Build history of the part. All positions in model axes, mm. Coordinates: 2 decimals unless noted, no trailing zeros. Order: outer loops, then holes, each group sorted by start corner. A loop starts at its lowest first (then second) coordinate and runs counter-clockwise, first axis right, second up. Notation, with made-up numbers: (42.5, 27) - (88.5, 27) arc R19 cw to (88.5, 49) - close; hole circle Ø9 at (48.5, 2). An arc over 180 degrees is marked (long way). Write each question's results on one line, items separated by ' | '.
from build123d import *

# Parameters (mm, degrees)
SKETCH1_W           = 2.87
SKETCH1_H           = 12.02
BOSS_EXTRUDE1_DEPTH = 2
CUT_EXTRUDE1_REACH  = 14.02


with BuildPart() as part:
    # Sketch1 → Boss-Extrude1 (new body)
    with BuildSketch(Plane.XY):
        with Locations((0, 6.01)):
            Rectangle(SKETCH1_W, SKETCH1_H)
    extrude(amount=BOSS_EXTRUDE1_DEPTH)

    # Sketch2 → Cut-Extrude1 (cut, up to next)
    with BuildSketch(Plane.XZ, mode=Mode.PRIVATE) as cut_extrude1_sk1:
        Polygon((0, -1.665063509), (1.25, 0.5), (-1.25, 0.5), align=None)
    cut_extrude1_tool1 = extrude(cut_extrude1_sk1.sketch, amount=-CUT_EXTRUDE1_REACH, mode=Mode.PRIVATE) & part.part
    add(cut_extrude1_tool1.solids().sort_by_distance((0, 0, -0.221688))[0], mode=Mode.SUBTRACT)


solid = part.part
1. Band-saw the part on A-A on z = 0.2. Give the cut face in (x, y) (3 decimals), then the cut area to 3 significant figures.
Solved:
outline: (-1.435, 0) - (-1.077, 0) - (-1.077, 12.02) - (-1.435, 12.02) - close; (1.077, 0) - (1.435, 0) - (1.435, 12.02) - (1.077, 12.02) - close | area: 8.61 mm2
2. Band-saw the part on B-B on y = 6.75. Give the cut face in (x, z) (3 decimals), then the cut area to 3 significant figures.
Solved:
outline: (-1.435, 0) - (-0.961, 0) - (-1.25, 0.5) - (1.25, 0.5) - (0.961, 0) - (1.435, 0) - (1.435, 2) - (-1.435, 2) - close | area: 4.63 mm2
3. Probe line 1 (Z direction, x = -0.3, y = 5.5); line 2 (Z direction, x = -1.1, y = 10.5); line 3 (X direction, y = 7.75, z = 0.1) (3 decimals). List the from-to ranges inside material, lowest first.
Solved:
line 1: z = 0.5 to 2 | line 2: z = 0 to 0.24, 0.5 to 2 | line 3: x = -1.435 to -1.019, 1.019 to 1.435
4. Two-plate mould, pull along Z, no slides. Class faces 1 (the face through (0, 0, 1)), 2 (the face through (0, 6, 0.5)), 3 (the face through (0, 6, 2)): +Z half, -Z half, draft (parallel to the pull), parting line (faces both ways), or undercut.
Solved:
face 1: draft | face 2: undercut | face 3: +Z half
5. Band-saw the part on C-C on x = -0.5. Give the cut face in (y, z).
Solved:
outline: (0, 0.5) - (12.02, 0.5) - (12.02, 2) - (0, 2) - close
